from build123d import *

# Parameters (mm, degrees)
F0_R      = 7.5
F1_DEPTH  = 15
F1_FACE_R = 7.5
F2_DEPTH  = 10
F2_TAPER  = 20


with BuildPart() as f1:
    # F0 (on Top) → F1 (new body)
    with BuildSketch(Plane.XY):
        Circle(F0_R)
    extrude(amount=F1_DEPTH)

    # F1_face (on face) → F2 (join)
    with BuildSketch(Plane.XY.offset(15)):
        Circle(F1_FACE_R)
    extrude(amount=F2_DEPTH, taper=F2_TAPER)

    # F3 (on Front) → F4 (revolve)
    with BuildSketch(Plane.XZ):
        with BuildLine():
            Line((0, 33), (0, 20))
            ThreePointArc((0, 20), (6.5, 26.5), (0, 33))
        make_face()
    revolve(axis=Axis((0, 0, 26.5), (0, 0, 1)))


solid = f1.part
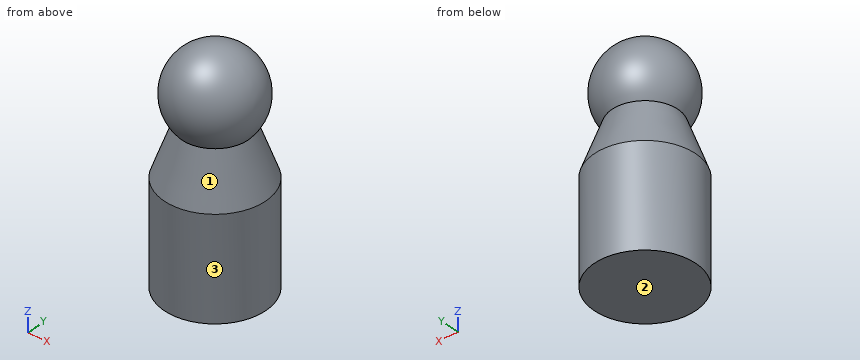
The listing builds one solid part. Answer for the finished solid, in the listing's coordinates (mm). Face numbers are marked on the shaded views. Coordinates: 2 decimals unless noted, no trailing zeros. Write each loop counter-clockwise with the first axis right and the second up, starting at its lowest first coordinate (ties: lowest second). Pieces come first, ordered by that corner, then holes. Notation, with made-up numbers: M 9,84.25 L 16,84.25 A14 ccw 16,90.25 Z; hole C 38,-17.75 d9. An arc over 180 degrees is marked long. Put each result on its own line as item: value. Start each with the question number.
1. Flat-ended cylindrical pins translate along their axes: P1, Ø1.5, axis at x = 4, z = 29, coming from the -Y side; P2, Ø8, axis at x = -3, z = 18.5, coming from the +Y side; P3, Ø6, axis at x = -0.5, z = 18.5, coming from the -Y side. Find the tip coordinate at first contact, or state that the pin passes through.
2. A cutting plane is placed at C-C on z = 18. Write down the section's boundary in (x, y).
3. A cutting plane is placed at A-A on y = 0. Write down the section's boundary in (x, z).
4. For a pull along Z with two mould halves and no side action, classify the marked faces 1, 2 and 3 as pulls with the +Z half, pulls with the -Z half, needs draft (parallel to the pull), parting line crosses it, or undercut.
5. Consider line 1 (Z direction, x = 5, y = 3.25); line 2 (Z direction, x = 4.75, y = 3); line 3 (X direction, y = 2.25, z = 15). Determine where each line is inside the solid, lowest interval first. Write a range as from..to.
Resolved:
1. P1: stops at y = -5.15
1. P2: stops at y = 7.42
1. P3: stops at y = -7.31
2. outline: C 0,0 d12.82
3. outline: M -7.5,0 L 7.5,0 L 7.5,15 L 4.88,22.2 A6.5 ccw long -4.88,22.2 L -7.5,15 Z
4. face 1: undercut
4. face 2: pulls with the -Z half
4. face 3: needs draft
5. line 1: z = 0..19.22, 23.91..29.09
5. line 2: z = 0..20.17, 23.23..29.77
5. line 3: x = -7.15..7.15
